Job drawing, mm, ordinate dimensions from the low corner. One solid piece. A direction names the side the tool comes from. Round coordinates to 2 decimals unless told otherwise and drop trailing zeros. Write each loop counter-clockwise with the first axis right and the second up, starting at its lowest first coordinate (ties: lowest second). Pieces come first, ordered by that corner, then holes.
1) Flat gauge pin, fed straight in: pin 1 (1.5 mm diameter, centred on x = 3.5, z = 23, fed in from +Y). Where does the tip first touch, or does it go through?
2) Saw through at A-A (x = 1). Write the cut outline in (y, z).
3) Saw through at C-C (z = 21.25). Write the cut outline in (x, y), plus the area to 3 significant figures.
4) Saw through at B-B (y = 4.75). Write the cut outline in (x, z).
5) Wall check: probe 1 along Z at (x, y) = (1.5, 7.5); probe 2 along Y at (x, z) = (4.75, 22); probe 3 along Y at (x, z) = (2.25, 19). Give the ranges that are in metal, low to high.
6) Which spindle directions (+Z, -Z, +X, -X, +Y, -Y) get a long thin tool onto all of the face, cutting with end or side? Do the marked faces 1 and 2. Say none if no direction does.
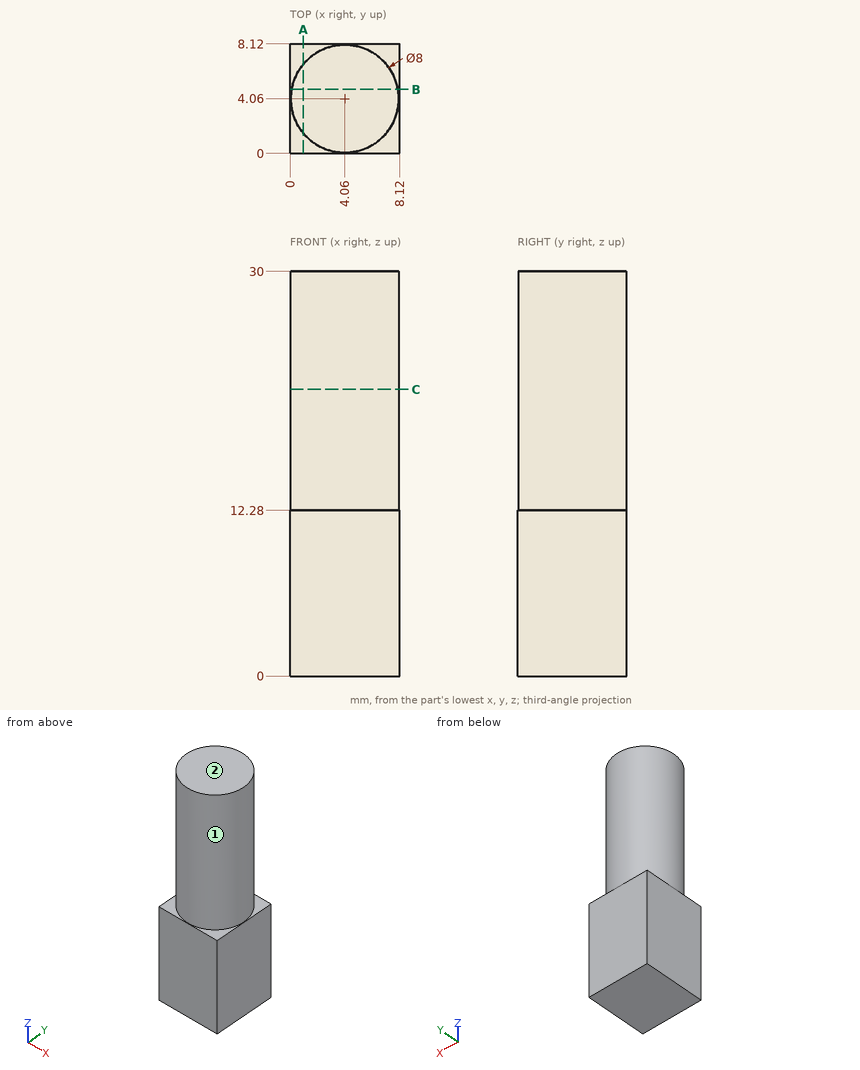
Evaluation:
1. pin 1: stops at y = 8.06
2. outline: (0, 0) - (8.12, 0) - (8.12, 12.28) - (6.64, 12.28) - (6.64, 30) - (1.48, 30) - (1.48, 12.28) - (0, 12.28) - close
3. outline: circle Ø8 at (4.06, 4.06)
3. area: 50.3 mm2
4. outline: (0, 0) - (8.12, 0) - (8.12, 12.28) - (8, 12.28) - (8, 30) - (0.12, 30) - (0.12, 12.28) - (0, 12.28) - close
5. probe 1: z = 0 to 12.28
5. probe 2: y = 0.12 to 8
5. probe 3: y = 0.49 to 7.63
6. face 1: +Z
6. face 2: +Z, +X, -X, +Y, -Y
